from build123d import *

# Parameters (mm, degrees)
F0_W      = 152.4
F0_H      = 152.4
F1_DEPTH  = 304.8
F2_R      = 28.56865
F3_DEPTH  = 25
F4_R      = 28.56865
F5_DEPTH  = 25
F6_R      = 20.6375
F7_DEPTH  = 264.16
F8_R      = 3.96875
F9_DEPTH  = 25.4
F10_R     = 3.96875
F11_DEPTH = 48.26


with BuildPart() as f1:
    # F0 (on Top) → F1 (new body)
    with BuildSketch(Plane.XY):
        with Locations((76.2, 76.2)):
            Rectangle(F0_W, F0_H)
    extrude(amount=F1_DEPTH)

    # F2 (on face) → F3 (cut)
    with BuildSketch(Plane.YZ.offset(152.4)):
        with Locations((76.2, 241.3)):
            Circle(F2_R)
    extrude(amount=-F3_DEPTH, mode=Mode.SUBTRACT)

    # F4 (on face) → F5 (cut)
    with BuildSketch(Plane(origin=(0, 0, 0), x_dir=(0, -1, 0), z_dir=(-1, 0, 0))):
        with Locations((-76.2, 241.3)):
            Circle(F4_R)
    extrude(amount=-F5_DEPTH, mode=Mode.SUBTRACT)

    # F6 (on face) → F7 (cut)
    with BuildSketch(Plane(origin=(25, 0, 0), x_dir=(0, -1, 0), z_dir=(-1, 0, 0))):
        with Locations((-76.2, 241.3)):
            Circle(F6_R)
    extrude(amount=-F7_DEPTH, mode=Mode.SUBTRACT)

    # F8 (on face) → F9 (cut)
    with BuildSketch(Plane(origin=(0, 0, 0), x_dir=(1, 0, 0), z_dir=(0, 0, -1))):
        with Locations((31.75, -31.75)):
            Circle(F8_R)
        with Locations((120.65, -31.75)):
            Circle(F8_R)
        with Locations((120.65, -120.65)):
            Circle(F8_R)
        with Locations((31.75, -120.65)):
            Circle(F8_R)
    extrude(amount=-F9_DEPTH, mode=Mode.SUBTRACT)

    # F10 (on face) → F11 (cut)
    with BuildSketch(Plane.XY.offset(304.8)):
        with Locations((76.2, 76.2)):
            Circle(F10_R)
    extrude(amount=-F11_DEPTH, mode=Mode.SUBTRACT)


solid = f1.part
Work out the finished part from the listing and answer in its coordinate system (mm). A direction names the side the tool comes from. Round coordinates to 2 decimals unless told otherwise and drop trailing zeros. Write each loop counter-clockwise with the first axis right and the second up, starting at its lowest first coordinate (ties: lowest second). Pieces come first, ordered by that corner, then holes. Notation, with made-up numbers: (13, -10) -> (49, -10) arc R12 ccw to (49, 11) -> close; hole circle Ø8 at (-6, 11). An arc over 180 degrees is marked (long way). Answer as CSV lines item,"result". Start each with the question number.
(1) The mould has two halves that part along X. Classify faces 1 (the cylindrical face through (12.325, 79.919, 269.626)), 2 (the flat face through (0, 75, 150)), 3 (the flat face through (152.4, 75, 150)), 4 (the cylindrical face through (79.985, 77.392, 283.478)): +X half, -X half, draft (parallel to the pull), parting line (faces both ways), or undercut.
(2) The part is cut by section A-A, the plane y = 76.2. Give the vertices of the cut face in (x, z), then the cut area to 3 significant figures.
(3) Find the intervals of material crossed by probe 1 along Y at (x, z) = (31.75, 14.25); probe 2 along X at (y, z) = (31, 11); probe 3 along Z at (x, y) = (96.5, 76.2), in increasing order.
(4) Each of these flat-tipped pins is pushed along its axis until it touches: pin 1 (17 mm diameter, centred on y = 62.5, z = 239, fed in from -X); pin 2 (4 mm diameter, centred on x = 120.5, y = 30, fed in from -Z). Where does it stop, or does it pass through?
(5) The part is cut by section C-C, the plane x = 76.2. Give the vertices of the cut face in (y, z) (1 decimal), then the cut area to 3 significant figures.
(6) The part is cut by section D-D, the plane z = 231.5. Give the vertices of the cut face in (x, y), then the cut area to 3 significant figures.
(7) The part is cut by section B-B, the plane x = 40. Give the vertices of the cut face in (y, z) (1 decimal).
(8) A tool of negligible diameter and unlimited length cuts with its end or side. For faces 5 (the flat face through (25, 68, 222)), 6 (the cylindrical face through (30.89, 35.624, 12.522)), 7 (the cylindrical face through (140.075, 72.481, 269.626)), 8 (the flat face through (75, 77, 0)), from which of +Z, -Z, +X, -X, +Y, -Y can it reach the whole face along a straight path? Write none if from no direction.
Output values:
1,face 1,"draft"
1,face 2,"-X half"
1,face 3,"+X half"
1,face 4,"undercut"
2,outline,"(0, 0) -> (152.4, 0) -> (152.4, 212.73) -> (127.4, 212.73) -> (127.4, 220.66) -> (25, 220.66) -> (25, 212.73) -> (0, 212.73) -> close; (0, 269.87) -> (25, 269.87) -> (25, 261.94) -> (72.23, 261.94) -> (72.23, 304.8) -> (0, 304.8) -> close; (80.17, 261.94) -> (127.4, 261.94) -> (127.4, 269.87) -> (152.4, 269.87) -> (152.4, 304.8) -> (80.17, 304.8) -> close"
2,area,"39,000 mm²"
3,probe 1,"y = 0 to 27.78, 35.72 to 116.68, 124.62 to 152.4"
3,probe 2,"x = 0 to 27.85, 35.65 to 116.75, 124.55 to 152.4"
3,probe 3,"z = 0 to 220.66, 261.94 to 304.8"
4,pin 1,"stops at x = 25"
4,pin 2,"stops at z = 25.4"
5,outline,"(0, 0) -> (152.4, 0) -> (152.4, 304.8) -> (80.2, 304.8) -> (80.2, 261.6) arc R20.6 cw (long way) to (72.2, 261.6) -> (72.2, 304.8) -> (0, 304.8) -> close"
5,area,"44,800 mm²"
6,outline,"(0, 0) -> (152.4, 0) -> (152.4, 49.36) -> (127.4, 49.36) -> (127.4, 58.04) -> (25, 58.04) -> (25, 49.36) -> (0, 49.36) -> close; (0, 103.04) -> (25, 103.04) -> (25, 94.36) -> (127.4, 94.36) -> (127.4, 103.04) -> (152.4, 103.04) -> (152.4, 152.4) -> (0, 152.4) -> close"
6,area,"16,800 mm²"
7,outline,"(0, 0) -> (152.4, 0) -> (152.4, 304.8) -> (0, 304.8) -> close; hole circle Ø41.3 at (76.2, 241.3)"
8,face 5,"-X"
8,face 6,"-Z"
8,face 7,"+X"
8,face 8,"-Z, +X, -X, +Y, -Y"
